Check sheet for the drawn part. Datum: minimum x, y, z corner. Units: mm. A direction names the side the tool comes from. Give positions to 0.01 mm unless a question says otherwise; leave off trailing zeros. Loops run counter-clockwise (first coordinate to the right, second up) from the corner with the lowest first, then second, coordinate; pieces in that order, holes last. Notation, with made-up numbers: (75.25, -2.5) -> (85.25, -2.5) arc R25 cw to (85.25, 33.5) -> close; hole circle Ø3 at (50, 76.5). An arc over 180 degrees is marked (long way). One line per question, with ' | ' between items.
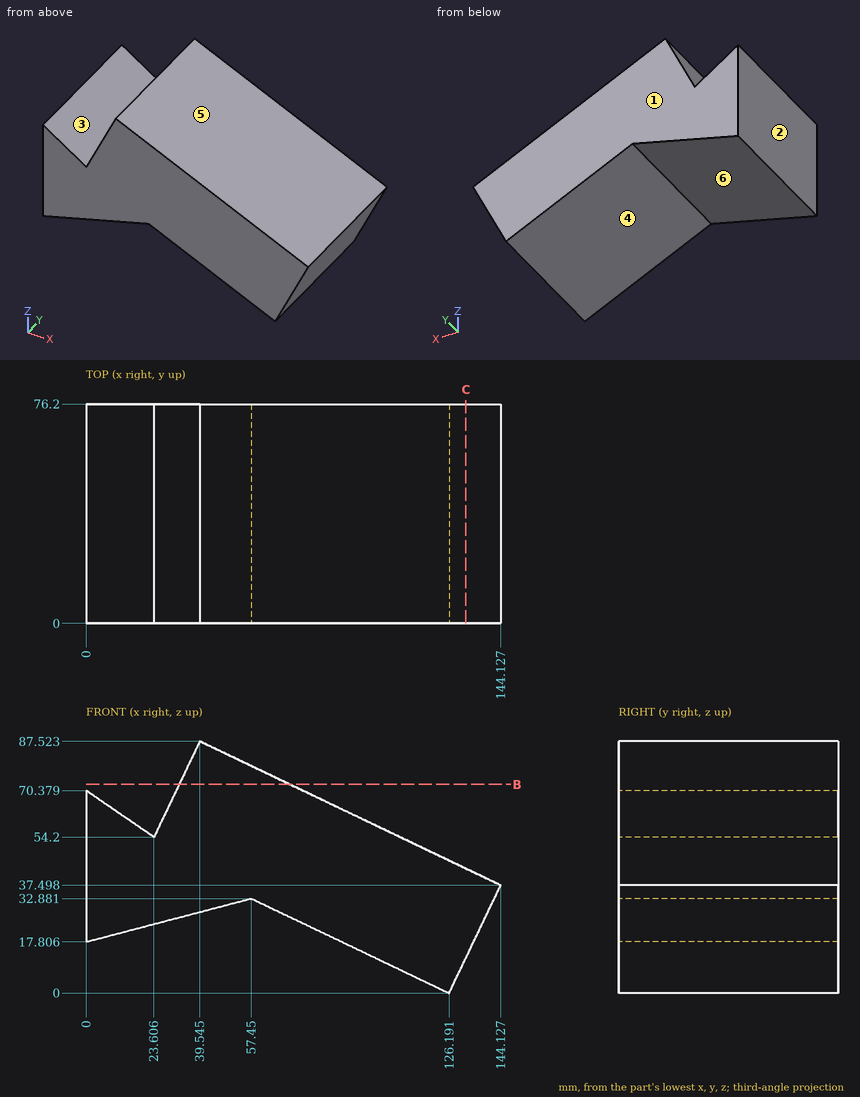
Item 1: Set-up check for the marked faces 5 and 6: record each of +Z, -Z, +X, -X, +Y, -Y from which the full face is reachable in a straight line by a thin tool's end or side.
Result:
face 5: +Z, +X, +Y, -Y | face 6: -Z, +Y, -Y
Item 2: Depth check by flat-ended pin: pin 1 Ø3 at (x, y) = (123.5, 39) entering from -Z; pin 2 Ø1 at (x, z) = (82.5, 19.5) entering from +Y. Enter the tip coordinate at first touch or a pass-through.
Result:
pin 1: z = 0.57 | pin 2: through
Item 3: Sectioned sample at C-C (x = 132). Record the cut outline in (y, z) (1 decimal).
Result:
outline: (0, 12.1) -> (76.2, 12.1) -> (76.2, 43.3) -> (0, 43.3) -> close
Item 4: Sectioned sample at B-B (z = 72.5). Record the cut outline in (x, y).
Result:
outline: (32.36, 0) -> (70.95, 0) -> (70.95, 76.2) -> (32.36, 76.2) -> close
Item 5: Release check for a two-part mould opening along X. For the marked faces 1, 2, 3 and 4 record: pulls with the +X half, pulls with the -X half, needs draft (parallel to the pull), parting line crosses it, or undercut.
Result:
face 1: needs draft | face 2: pulls with the -X half | face 3: undercut | face 4: undercut
Item 6: Scan lines: probe 1 along X at (y, z) = (25.5, 59) (1 decimal); probe 2 along X at (y, z) = (23, 64.5) (1 decimal); probe 3 along X at (y, z) = (21.5, 4) (1 decimal). Record each from-to range of solid material in increasing order.
Result:
probe 1: 0 to 16.6, 25.9 to 99.2 | probe 2: 0 to 8.6, 28.5 to 87.7 | probe 3: 117.8 to 128.1
